Verification items for the finished model (mm, model axes). Face numbers are marked on the shaded views. A direction names the side the tool comes from. Round coordinates to 2 decimals unless told otherwise and drop trailing zeros. Write each loop counter-clockwise with the first axis right and the second up, starting at its lowest first coordinate (ties: lowest second). Pieces come first, ordered by that corner, then holes. Notation, with made-up numbers: (-5, -32.5) - (13, -32.5) arc R15 ccw to (13, -22.5) - close; hole circle Ø2 at (55, 78.25). An arc over 180 degrees is marked (long way). Answer as a JSON object with one key per item and string values. Group by question number.
1) Mould release check, pull along Z, two halves, no side actions. Record for the marked faces 1, 2, 3 and 4: +Z half, -Z half, draft (parallel to the pull), parting line (faces both ways), or undercut.
2) Go/stop test with flat-tipped pins: pin 1 Ø3.5 at (x, y) = (0, 35.5) entering from -Z; pin 2 Ø3.5 at (x, z) = (0, -35) entering from +Y. Record where each tip stops, or that it passes through.
3) Section check A-A (z = -35). Enter the section's corners in (x, y), then the cut area to 3 significant figures.
4) Thickness scan on line 1 (Z direction, x = -1.5, y = 5); line 2 (Y direction, x = 0, z = -54.85); line 3 (Y direction, x = -11.25, z = -28). Record the ranges inside material, lowest first.
5) Set-up check for the marked faces 5 and 6: record each of +Z, -Z, +X, -X, +Y, -Y from which the full face is reachable in a straight line by a thin tool's end or side.
6) Section check D-D (z = -28). Enter the section's corners in (x, y), then the cut area to 3 significant figures.
7) Section check B-B (y = 21). Enter the section's corners in (x, z).
8) Section check C-C (y = 35.5). Enter the section's corners in (x, z), then the cut area to 3 significant figures.
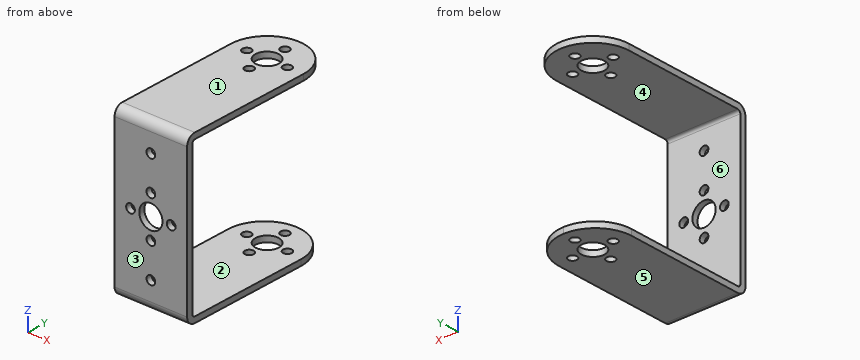
```python
from build123d import *

# Parameters (mm, degrees)
BASE_FLANGE1_DEPTH           = 2
EDGE_FLANGE1_DEPTH           = 25
EDGE_FLANGE2_STRIP_W         = 10
EDGE_FLANGE2_STRIP_H         = 2
EDGE_FLANGE2_STRIP_CUT_DEPTH = 25
EDGE_FLANGE2_DEPTH           = 25
CUT_EXTRUDE1_DEPTH           = 2
SKETCH19_R                   = 4
CUT_EXTRUDE2_DEPTH           = 80.481129836
M3X0_5_TAPPED_HOLE1_D        = 3
SKETCH22_R                   = 4
CUT_EXTRUDE3_DEPTH           = 81.176368089
M3X0_5_TAPPED_HOLE2_D        = 3


# Sheet-metal steps are written as plain solids
with BuildPart() as part:
    # Sketch8 → Base-Flange1 (new body)
    with BuildSketch(Plane.XY):
        with BuildLine():
            Line((-12.5, 0), (12.5, 0))
            Line((12.5, 0), (12.5, 42.5))
            ThreePointArc((12.5, 42.5), (0, 55), (-12.5, 42.5))
            Line((-12.5, 42.5), (-12.5, 0))
        make_face()
    extrude(amount=-BASE_FLANGE1_DEPTH)

    # Edge-Flange1 section (across the edge) → Edge-Flange1 (add)
    with BuildSketch(Plane(origin=(12.5, -1, -2), x_dir=(0, 1, 0), z_dir=(-1, 0, 0))):
        with BuildLine():
            Line((-2, 1), (-2, 52))
            Line((-2, 52), (0, 52))
            Line((0, 52), (0, 1))
            ThreePointArc((0, 1), (0.292893219, 0.292893219), (1, 0))
            Line((1, 0), (1, -2))
            ThreePointArc((1, -2), (-1.121320344, -1.121320344), (-2, 1))
        make_face()
    extrude(amount=EDGE_FLANGE1_DEPTH)

    # Edge-Flange2 strip (across the edge) → Edge-Flange2 strip cut (cut)
    with BuildSketch(Plane(origin=(12.5, -1, -54), x_dir=(0, 0, 1), z_dir=(-1, 0, 0))):
        with Locations((-4, -1)):
            Rectangle(EDGE_FLANGE2_STRIP_W, EDGE_FLANGE2_STRIP_H)
    extrude(amount=EDGE_FLANGE2_STRIP_CUT_DEPTH, mode=Mode.SUBTRACT)

    # Edge-Flange2 section (across the edge) → Edge-Flange2 (add)
    with BuildSketch(Plane(origin=(12.5, -1, -54), x_dir=(0, 0, 1), z_dir=(-1, 0, 0))):
        with BuildLine():
            Line((-2, 1), (-2, 55))
            Line((-2, 55), (0, 55))
            Line((0, 55), (0, 1))
            ThreePointArc((0, 1), (0.292893219, 0.292893219), (1, 0))
            Line((1, 0), (1, -2))
            ThreePointArc((1, -2), (-1.121320344, -1.121320344), (-2, 1))
        make_face()
    extrude(amount=EDGE_FLANGE2_DEPTH)

    # Sketch18 → Cut-Extrude1 (cut)
    with BuildSketch(Plane(origin=(0, 0, -56), x_dir=(-1, 0, 0), z_dir=(0, 0, -1))):
        with BuildLine():
            ThreePointArc((0, 54), (8.838834765, 50.338834765), (12.5, 41.5))
            Line((12.5, 41.5), (12.5, 54))
            Line((12.5, 54), (0, 54))
        make_face()
        with BuildLine():
            ThreePointArc((-12.5, 41.5), (-8.838834765, 50.338834765), (0, 54))
            Line((0, 54), (-12.5, 54))
            Line((-12.5, 54), (-12.5, 41.5))
        make_face()
    extrude(amount=-CUT_EXTRUDE1_DEPTH, mode=Mode.SUBTRACT)

    # Sketch19 → Cut-Extrude2 (cut, through all)
    with BuildSketch(Plane.XY):
        with Locations((0, 42.5)):
            Circle(SKETCH19_R)
    extrude(amount=-CUT_EXTRUDE2_DEPTH, mode=Mode.SUBTRACT)

    # M3x0.5 Tapped Hole1 (through all)
    with Locations(Plane.XY):
        with Locations((0, 49.5), (-7, 42.5), (0, 35.5), (7, 42.5)):
            Hole(M3X0_5_TAPPED_HOLE1_D / 2)

    # Sketch22 → Cut-Extrude3 (cut, through all)
    with BuildSketch(Plane(origin=(0, -1, 0), x_dir=(1, 0, 0), z_dir=(0, 1, 0))):
        with Locations(Location((0, 28, 0), (0, 0, 270))):
            Circle(SKETCH22_R)
    extrude(amount=-CUT_EXTRUDE3_DEPTH, mode=Mode.SUBTRACT)

    # M3x0.5 Tapped Hole2 (through all)
    with Locations(Plane(origin=(0, -1, 0), x_dir=(1, 0, 0), z_dir=(0, 1, 0))):
        with Locations((7, 28), (-7, 28), (0, 35), (0, 21), (0, 9.4), (0, 46.6)):
            Hole(M3X0_5_TAPPED_HOLE2_D / 2)


solid = part.part
```
Returned:
{
 "1": {"face 1": "+Z half", "face 2": "undercut", "face 3": "draft", "face 4": "undercut"},
 "2": {"pin 1": "z = -56", "pin 2": "y = -1"},
 "3": {"outline": "(-12.5, -3) - (-1.5, -3) - (-1.5, -1) - (-12.5, -1) - close; (1.5, -3) - (12.5, -3) - (12.5, -1) - (1.5, -1) - close", "area": "44.0 mm2"},
 "4": {"line 1": "-56 to -54, -2 to 0", "line 2": "-2.36 to 34, 37 to 38.5, 46.5 to 48, 51 to 54", "line 3": "-3 to -1"},
 "5": {"face 5": "-Z, +X, -X, +Y, -Y", "face 6": "+X, -X, +Y"},
 "6": {"outline": "(-12.5, -3) - (-8.5, -3) - (-8.5, -1) - (-12.5, -1) - close; (-5.5, -3) - (-4, -3) - (-4, -1) - (-5.5, -1) - close; (4, -3) - (5.5, -3) - (5.5, -1) - (4, -1) - close; (8.5, -3) - (12.5, -3) - (12.5, -1) - (8.5, -1) - close", "area": "22.0 mm2"},
 "7": {"outline": "(-12.5, -56) - (12.5, -56) - (12.5, -54) - (-12.5, -54) - close; (-12.5, -2) - (12.5, -2) - (12.5, 0) - (-12.5, 0) - close"},
 "8": {"outline": "(-12.5, -56) - (-1.5, -56) - (-1.5, -54) - (-12.5, -54) - close; (-12.5, -2) - (-1.5, -2) - (-1.5, 0) - (-12.5, 0) - close; (1.5, -56) - (12.5, -56) - (12.5, -54) - (1.5, -54) - close; (1.5, -2) - (12.5, -2) - (12.5, 0) - (1.5, 0) - close", "area": "88.0 mm2"}
}
